from build123d import *

# Parameters (mm, degrees)
BOSS_EXTRUDE1_DEPTH                          = 12
SKETCH2_R                                    = 4.75
CUT_EXTRUDE1_DEPTH                           = 35
SKETCH3_R                                    = 2.05
CUT_EXTRUDE2_DEPTH                           = 35
SKETCH4_W                                    = 5.9
SKETCH4_H                                    = 8.15
CSK_FOR_M3_CROSS_COUNTERSUNK_HEAD_SC_2_COUNT = 2
CSK_FOR_M3_CROSS_COUNTERSUNK_HEAD_SC_2_PITCH = 36


with BuildPart() as part:
    # Sketch1 → Boss-Extrude1 (new body)
    with BuildSketch(Plane.XY):
        with BuildLine():
            Line((-9.1, 0), (-25, 0))
            ThreePointArc((-25, 0), (0, -25), (25, 0))
            Line((25, 0), (9.211282306, 0))
            Line((9.211282306, 0), (9.1, 0))
            Line((9.1, 0), (-9.1, 0))
        make_face()
    extrude(amount=BOSS_EXTRUDE1_DEPTH)

    # Sketch2 → Cut-Extrude1 (cut)
    with BuildSketch(Plane(origin=(0, -40, 0), x_dir=(1, 0, 0), z_dir=(0, 1, 0))):
        with Locations((18, -6)):
            Circle(SKETCH2_R)
        with Locations((-18, -6)):
            Circle(SKETCH2_R)
    extrude(amount=CUT_EXTRUDE1_DEPTH, mode=Mode.SUBTRACT)

    # Sketch3 → Cut-Extrude2 (cut)
    with BuildSketch(Plane.XZ.offset(5)):
        with Locations((18, 6)):
            Circle(SKETCH3_R)
        with Locations((-18, 6)):
            Circle(SKETCH3_R)
    extrude(amount=-CUT_EXTRUDE2_DEPTH, mode=Mode.SUBTRACT)

    # Sketch4 → Cut-Revolve1 (revolve, cut)
    with BuildSketch(Plane(origin=(0, 0, 0), x_dir=(1, 0, 0), z_dir=(0, 1, 0))):
        Polygon((0, -12), (0, 0), (-7.2, 0), (-7.2, -1.925), (-7.2, -10.075), (-7.2, -12), align=None)
        with Locations((-10.15, -6)):
            Rectangle(SKETCH4_W, SKETCH4_H)
    revolve(axis=Axis((0, 0, 0), (0, 0, 1)), mode=Mode.SUBTRACT)

    # Sketch6 → CSK for M3 Cross Countersunk Head Screw1 (revolve, cut)
    with BuildSketch(Plane(origin=(18, 0, 6), x_dir=(0, 0, 1), z_dir=(1, 0, 0))):
        Polygon((0, 0), (0, 25), (2.5, 25), (2.5, 2.860133251), (2.7, 0), align=None)
    csk_for_m3_cross_countersunk_head_screw1 = revolve(axis=Axis((18, 6.35, 6), (0, -1, 0)), mode=Mode.SUBTRACT)

    # CSK for M3 Cross Countersunk Head Sc 2: CSK for M3 Cross Countersunk Head Screw1 ×2
    with Locations(*[(-i * CSK_FOR_M3_CROSS_COUNTERSUNK_HEAD_SC_2_PITCH, 0, 0) for i in range(1, CSK_FOR_M3_CROSS_COUNTERSUNK_HEAD_SC_2_COUNT)]):
        add(csk_for_m3_cross_countersunk_head_screw1, mode=Mode.SUBTRACT)


solid = part.part
The listing builds one solid part. Answer for the finished solid, in the listing's coordinates (mm). A direction names the side the tool comes from. Coordinates: 2 decimals unless noted, no trailing zeros. Loops run counter-clockwise (first coordinate to the right, second up) from the corner with the lowest first, then second, coordinate; pieces in that order, holes last.
1) Flat-ended cylindrical pins translate along their axes: pin 1 Ø1 at (x, z) = (-6.5, 6) entering from +Y; pin 2 Ø5 at (x, z) = (20, 5.5) entering from -Y; pin 3 Ø4 at (x, z) = (18, 6) entering from -Y; pin 4 Ø6 at (y, z) = (-11, 4) entering from +X. Find the tip coordinate at first contact, or state that the pin passes through.
2) Find section A-A on y = -2.25. Write down the section's boundary in (x, z) (3 decimals), then the cut area to 3 significant figures.
3) Find the intervals of material crossed by L1, parallel to Z at x = -5.5, y = -7.5 (3 decimals); L2, parallel to X at y = -7.5, z = 9.5; L3, parallel to X at y = -7.75, z = 5.25, in increasing order.
4) Find section D-D on x = 0. Write down the section's boundary in (y, z) (3 decimals).
5) A tool of negligible diameter and unlimited length cuts with its end or side. For faces 5 (the face through (0, -8, 1.925)), 6 (the face through (-13.47, -11.41, 4.57)), 7 (the face through (-0.16, -7.2, 0.98)), from which of +Z, -Z, +X, -X, +Y, -Y can it reach the whole face along a straight path? Write none if from no direction.
6) Find section C-C on z = 6. Write down the section's boundary in (x, y), then the cut area to 3 significant figures.
7) Determine the mould class of faces 1 (the face through (-0.16, -7.2, 11.05)), 2 (the face through (0, -12, 12)), 3 (the face through (-20.11, -3.92, 7.34)), 4 (the face through (-16, -5, 8)) for opening direction Z: pulls with the +Z half, pulls with the -Z half, needs draft (parallel to the pull), parting line crosses it, or undercut.
8) Find section B-B on x = 18. Write down the section's boundary in (y, z).
Values:
1. pin 1: stops at y = -11.07
1. pin 2: stops at y = -5
1. pin 3: passes through
1. pin 4: stops at x = 23.69
2. outline: (-24.899, 0) - (-6.839, 0) - (-6.839, 1.925) - (-12.905, 1.925) - (-12.905, 10.075) - (-6.839, 10.075) - (-6.839, 12) - (-24.899, 12) - close; (6.839, 0) - (24.899, 0) - (24.899, 12) - (6.839, 12) - (6.839, 10.075) - (12.905, 10.075) - (12.905, 1.925) - (6.839, 1.925) - close; hole circle Ø5.085 at (-18, 6); hole circle Ø5.085 at (18, 6)
2. area: 294 mm2
3. L1: z = 0 to 1.925, 10.075 to 12
3. L2: x = -23.85 to -21.21, -14.79 to -10.74, 10.74 to 14.79, 21.21 to 23.85
3. L3: x = -23.77 to -22.69, -13.31 to -10.56, 10.56 to 13.31, 22.69 to 23.77
4. outline: (-25, 0) - (-7.2, 0) - (-7.2, 1.925) - (-13.1, 1.925) - (-13.1, 10.075) - (-7.2, 10.075) - (-7.2, 12) - (-25, 12) - close
5. face 5: +Y
5. face 6: -Y
5. face 7: +Z, -Z, +Y
6. outline: (-25, 0) arc R25 ccw to (-22.75, -10.37) - (-22.75, -5) - (-20.5, -5) - (-20.5, -2.86) - (-20.7, 0) - close; (-15.5, -5) - (-13.25, -5) - (-13.25, -21.2) arc R25 ccw to (13.25, -21.2) - (13.25, -5) - (15.5, -5) - (15.5, -2.86) - (15.3, 0) - (13.1, 0) arc R13.1 cw to (-13.1, 0) - (-15.3, 0) - (-15.5, -2.86) - close; (20.5, -5) - (22.75, -5) - (22.75, -10.37) arc R25 ccw to (25, 0) - (20.7, 0) - (20.5, -2.86) - close
6. area: 436 mm2
7. face 1: needs draft
7. face 2: pulls with the +Z half
7. face 3: undercut
7. face 4: undercut
8. outline: (-17.35, 0) - (0, 0) - (0, 3.3) - (-2.86, 3.5) - (-5, 3.5) - (-5, 1.25) - (-17.35, 1.25) - close; (-17.35, 10.75) - (-5, 10.75) - (-5, 8.5) - (-2.86, 8.5) - (0, 8.7) - (0, 12) - (-17.35, 12) - close
